```python
from build123d import *
from OCP.BRepFilletAPI import BRepFilletAPI_MakeChamfer

# Parameters (mm, degrees)
BOSS_EXTRUDE1_DEPTH = 2.3749
CHAMFER1_SIZE       = 2.3749
CHAMFER1_SIZE2      = 13.468727193
CHAMFER2_SIZE       = 2.3749
CHAMFER2_SIZE_2     = 13.468727193


with BuildPart() as part:
    # Sketch1 → Boss-Extrude1 (new, symmetric)
    with BuildSketch(Plane(origin=(0, 0, 0), x_dir=(1, 0, 0), z_dir=(0, 1, 0))):
        Polygon((-101.6, 0), (58.248479739, 190.5), (185.248479739, 190.5), (101.6, 0), (101.6, -22.225), (-101.6, -22.225), align=None)
    extrude(amount=BOSS_EXTRUDE1_DEPTH, both=True)

    # Chamfer1: one chamfer whose edges measure the first distance from different faces: ONE call of the kernel's chamfer builder (chamfer() names one face for all edges)
    chamfer1_edges_1 = [part.edges().sort_by_distance(p)[0] for p in [
        (121.748479739, 2.3749, -190.5),
    ]]
    chamfer1_side_1 = [part.faces().sort_by_distance(p)[0] for p in [
        (121.748479739, 0, -190.5),
    ]]
    chamfer1_edges_2 = [part.edges().sort_by_distance(p)[0] for p in [
        (-21.67576013, 2.3749, -95.25),
    ]]
    chamfer1_side_2 = [part.faces().sort_by_distance(p)[0] for p in [
        (-21.67576013, 0, -95.25),
    ]]
    chamfer1_edges_3 = [part.edges().sort_by_distance(p)[0] for p in [
        (143.42423987, 2.3749, -95.25),
    ]]
    chamfer1_side_3 = [part.faces().sort_by_distance(p)[0] for p in [
        (143.42423987, 0, -95.25),
    ]]
    chamfer1 = BRepFilletAPI_MakeChamfer(part.part.solid().wrapped)
    for e in chamfer1_edges_1:
        chamfer1.Add(CHAMFER1_SIZE, CHAMFER1_SIZE2, e.wrapped, chamfer1_side_1[0].wrapped)  # the first distance lies on this face
    for e in chamfer1_edges_2:
        chamfer1.Add(CHAMFER1_SIZE, CHAMFER1_SIZE2, e.wrapped, chamfer1_side_2[0].wrapped)  # the first distance lies on this face
    for e in chamfer1_edges_3:
        chamfer1.Add(CHAMFER1_SIZE, CHAMFER1_SIZE2, e.wrapped, chamfer1_side_3[0].wrapped)  # the first distance lies on this face
    add(Compound.cast(chamfer1.Shape()), mode=Mode.REPLACE)

    # Chamfer2
    # the kernel refuses this chamfer: 13.468727193, 2.3749 mm, written as the material it takes off along each edge
    with BuildSketch(Plane(origin=(199.319755492, -2.3749, -222.545747147), x_dir=(0.19240697277850308, 0.9776715712462557, 0.08448583078297824), z_dir=(-0.40204782056593685, 0, 0.9156186706146726))) as chamfer2_piece_1_section:
        Polygon((CHAMFER2_SIZE * 0.977671571246, CHAMFER2_SIZE * 0.210138760767), (-CHAMFER2_SIZE_2 * 0.210138760774, CHAMFER2_SIZE_2 * 0.977671571276), (0, 0), align=None)
    chamfer2_piece_1 = extrude(amount=278.054066026, mode=Mode.PRIVATE)
    chamfer2_piece_1 = split(chamfer2_piece_1, bisect_by=Plane(origin=(101.6, -1.721128259, -118.063928537), z_dir=(1, 0, 0)), keep=Keep.TOP, mode=Mode.PRIVATE)
    add(chamfer2_piece_1, mode=Mode.SUBTRACT)
    with BuildSketch(Plane(origin=(-124.096930076, -2.3749, 26.81079724), x_dir=(-0.1609756299698045, 0.9776715712462571, -0.13507459173619368), z_dir=(0.6427876096865406, 0, -0.7660444431189771))) as chamfer2_piece_2:
        Polygon((CHAMFER2_SIZE * 0.977671571246, CHAMFER2_SIZE * 0.210138760767), (-CHAMFER2_SIZE_2 * 0.210138760774, CHAMFER2_SIZE_2 * 0.977671571276), (0, 0), align=None)
    extrude(amount=318.678108919, mode=Mode.SUBTRACT)
    with BuildSketch(Plane(origin=(23.249469589, -2.3749, -190.5), x_dir=(0, 0.977671571246258, -0.21013876076743496), z_dir=(1, 0, 0))) as chamfer2_piece_3:
        Polygon((CHAMFER2_SIZE * 0.977671571246, CHAMFER2_SIZE * 0.210138760767), (-CHAMFER2_SIZE_2 * 0.210138760774, CHAMFER2_SIZE_2 * 0.977671571276), (0, 0), align=None)
    extrude(amount=196.998020301, mode=Mode.SUBTRACT)


solid = part.part
```
Source: CAD feature listing. Evaluate the final solid. Frame: model axes, mm. Coordinates: 2 decimals unless noted, no trailing zeros. Loops run counter-clockwise (first coordinate to the right, second up) from the corner with the lowest first, then second, coordinate; pieces in that order, holes last. Notation, with made-up numbers: M 72.5,72 L 87.5,72 A26 cw 87.5,107 Z; hole C 53.25,41 d10. An arc over 180 degrees is marked long. Put each result on its own line as item: value. Start each with the question number.
1) Cut plane A-A on z = -87. Return the cut outline in (x, y), then the cut area to 3 significant figures.
2) Ray query, L1, parallel to Y at x = 160, z = -181; L2, parallel to Y at x = 114, z = -48.5. Return the intervals inside material, ascending. Write a range as from..to.
3) Contact query for flat-ended pins moving along their axis: pin 1 Ø12 at (x, z) = (-59.5, -44) entering from +Y; pin 2 Ø2 at (y, z) = (-0.5, -131) entering from -X. Output: stop coordinate, or through.
4) Cut plane B-B on y = 1.45. Return the cut outline in (x, z) (3 decimals).
5) Cut plane C-C on x = -26. Return the cut outline in (y, z) (3 decimals).
6) Cut plane D-D on x = -56. Return the cut outline in (y, z) (3 decimals).
The answers:
1. outline: M -28.6,0 L -11.02,-2.37 L 125.09,-2.37 L 139.8,0 L 125.09,2.37 L -11.02,2.37 Z
1. area: 723 mm²
2. L1: y = -1.68..1.68
2. L2: y = -1.44..1.44
3. pin 1: stops at y = 1.76
3. pin 2: stops at x = 7.6
4. outline: M -101.6,12.793 L 62.083,-182.277 L 172.656,-182.277 L 101.6,-20.454 L 101.6,22.225 L -101.6,22.225 Z
5. outline: M -2.375,-69.143 L 0,-90.097 L 2.375,-69.143 L 2.375,22.225 L -2.375,22.225 Z
6. outline: M -2.375,-33.39 L 0,-54.344 L 2.375,-33.39 L 2.375,22.225 L -2.375,22.225 Z
